Verification items for the finished model (mm, model axes). A direction names the side the tool comes from. Coordinates: 2 decimals unless noted, no trailing zeros. Write each loop counter-clockwise with the first axis right and the second up, starting at its lowest first coordinate (ties: lowest second). Pieces come first, ordered by that corner, then holes. Notation, with made-up numbers: (83, 36) - (113, 36) arc R26 ccw to (113, 65) - close; hole circle Ø6 at (81.25, 45.5). An arc over 180 degrees is marked (long way). Answer as CSV lines item,"result". Start each with the question number.
```python
from build123d import *

# Parameters (mm, degrees)
F0_W     = 88.9
F0_H     = 38.1
F1_DEPTH = 50.8
F2_W     = 38.1
F2_H     = 25.4
F3_DEPTH = 38.101
F4_W     = 63.5
F4_H     = 25.4
F5_DEPTH = 50.801
F6_R     = 6.35
F6_R_2   = 6.637383
F7_DEPTH = 12.701


with BuildPart() as f1:
    # F0 (on Front) → F1 (new body)
    with BuildSketch(Plane.XZ):
        Rectangle(F0_W, F0_H)
    extrude(amount=F1_DEPTH)

    # F2 (on face) → F3 (cut, through all)
    with BuildSketch(Plane.XY.offset(19.05)):
        with Locations((25.4, -38.1)):
            Rectangle(F2_W, F2_H)
    extrude(amount=-F3_DEPTH, mode=Mode.SUBTRACT)

    # F4 (on face) → F5 (cut, through all)
    with BuildSketch(Plane.XZ.offset(50.8)):
        with Locations((0, 6.35)):
            Rectangle(F4_W, F4_H)
    extrude(amount=-F5_DEPTH, mode=Mode.SUBTRACT)

    # F6 (on face) → F7 (cut, through all)
    with BuildSketch(Plane.XY.offset(-6.35)):
        with Locations((-19.05, -38.1)):
            Circle(F6_R)
        with Locations((6.35, -12.7)):
            Circle(F6_R_2)
    extrude(amount=-F7_DEPTH, mode=Mode.SUBTRACT)


solid = f1.part
```
1. Cross-section at D-D (z = -14). Record the cut outline in (x, y).
2. Draft check along X on faces 4 (the face through (6.35, -38, -13)), 5 (the face through (12.5, -15.2, -12.6)), 6 (the face through (-31.75, -26, 6)), 7 (the face through (-11, -19, -19.05)). Enter one of: pulls with the +X half, pulls with the -X half, needs draft (parallel to the pull), parting line crosses it, or undercut.
3. Cross-section at C-C (z = 15). Record the cut outline in (x, y), and give its area (3 significant figures).
4. Depth check by flat-ended pin: P1, Ø20.5, axis at x = -19.05, y = -38.1, coming from the +Z side; P2, Ø7.5, axis at y = -35.5, z = 12, coming from the +X side; P3, Ø6.5, axis at y = -36, z = -13, coming from the +X side. Enter the tip coordinate at first touch or a pass-through.
5. Cross-section at A-A (x = 10.5). Record the cut outline in (y, z), and give its area (3 significant figures).
6. Access from +Z, -Z, +X, -X, +Y, -Y to the whole of each face (thin tool, end or side, straight path). Record for faces 1 (the face through (34, -25.4, -4)), 2 (the face through (-25.394, -37.821, -12.611)), 3 (the face through (31.75, -13, 6)).
7. Cross-section at B-B (y = -38.1). Record the cut outline in (x, z).
8. Scan lines: line 1 along Y through (x, z) = (-19.05, -12); line 2 along X through (y, z) = (-7, 5.5); line 3 along X through (y, z) = (-37, -5). Record each from-to range of solid material in increasing order. Write a range as from..to.
Completed:
1,outline,"(-44.45, -50.8) - (6.35, -50.8) - (6.35, -25.4) - (44.45, -25.4) - (44.45, 0) - (-44.45, 0) - close; hole circle Ø12.7 at (-19.05, -38.1); hole circle Ø13.27 at (6.35, -12.7)"
2,face 4,"pulls with the +X half"
2,face 5,"undercut"
2,face 6,"undercut"
2,face 7,"needs draft"
3,outline,"(-44.45, -50.8) - (-31.75, -50.8) - (-31.75, 0) - (-44.45, 0) - close; (31.75, -25.4) - (44.45, -25.4) - (44.45, 0) - (31.75, 0) - close"
3,area,"968 mm2"
4,P1,"stops at z = -6.35"
4,P2,"stops at x = -31.75"
4,P3,"stops at x = 6.35"
5,outline,"(-25.4, -19.05) - (-17.88, -19.05) - (-17.88, -6.35) - (-25.4, -6.35) - close; (-7.52, -19.05) - (0, -19.05) - (0, -6.35) - (-7.52, -6.35) - close"
5,area,"191 mm2"
6,face 1,"+Z, -Z, +X, -Y"
6,face 2,"+Z, -Z"
6,face 3,"+Z, +Y, -Y"
7,outline,"(-44.45, -19.05) - (-25.4, -19.05) - (-25.4, -6.35) - (-31.75, -6.35) - (-31.75, 19.05) - (-44.45, 19.05) - close; (-12.7, -19.05) - (6.35, -19.05) - (6.35, -6.35) - (-12.7, -6.35) - close"
8,line 1,"y = -50.8..-44.45, -31.75..0"
8,line 2,"x = -44.45..-31.75, 31.75..44.45"
8,line 3,"x = -44.45..-31.75"
